Source: CAD feature listing. Evaluate the final solid. Frame: model axes, mm. A direction names the side the tool comes from. Give positions to 0.01 mm unless a question says otherwise; leave off trailing zeros. Write each loop counter-clockwise with the first axis right and the second up, starting at its lowest first coordinate (ties: lowest second). Pieces come first, ordered by that corner, then holes. Notation, with made-up numbers: (39, 79.5) - (68, 79.5) arc R29 ccw to (68, 99.5) - close; hole circle Ø1 at (71.25, -7.5). An arc over 180 degrees is marked (long way). Answer as a JSON object with one key per item and string values. Group by question number.
from build123d import *

# Parameters (mm, degrees)
F0_W        = 0.4
F0_H        = 28.4
F1_DEPTH    = 5
F2_T1_DEPTH = 17.9903810568
F3_T1_DEPTH = 29.4948974279
F3_T3_DEPTH = 30


# Not quite as in the source:
# - a fillet or chamfer that OpenCascade refuses, or shapes differently, is made with other operations: its cross-section is extruded or revolved along the edge and cut away or added


with BuildPart() as f1:
    # F0 (on Top) → F1 (new body)
    with BuildSketch(Plane.XY):
        Polygon((-17.5608190332, -5.5), (-10.5608190332, -5.5), (-11.8766345504, -2.5), (-14.2008190332, -2.5), (-14.2008190332, -0.1), (-14.2008190332, 0), (0, 0), (0, 28.4), (-6.4, 28.4), (-6.4, 26.9), (-2.4, 26.9), (-2.4, 2.7), (-12.7, 2.7), (-13.5608190332, 5.2), (-17.5608190332, 5.2), align=None)
        Polygon((-14.2008190332, 0), (-14.2008190332, -0.1), (0.4, -0.1), (0.4, 0), (0, 0), align=None)
        with Locations((0.2, 14.2)):
            Rectangle(F0_W, F0_H)
    extrude(amount=F1_DEPTH)

    # F2: fillet of radius 3 on 1 edges, made by hand

    # F2_s2 → F2_t1 (cut)
    with BuildSketch(Plane.XY.offset(-6.4951905284)):
        with BuildLine():
            ThreePointArc((-3.8019237886, 28.4), (-5.3019237886, 27.9980762114), (-6.4, 26.9))
            Line((-6.4, 26.9), (-6.4, 28.4))
            Line((-6.4, 28.4), (-3.8019237886, 28.4))
        make_face()
    extrude(amount=F2_T1_DEPTH, mode=Mode.SUBTRACT)

    # F3: fillet of radius 5 on 2 edges, made by hand

    # F3_s2 → F3_t1 (cut)
    with BuildSketch(Plane.XY.offset(-12.2474487139)):
        with BuildLine():
            ThreePointArc((-17.5608190332, 0.3010205144), (-16.4338023794, 3.4632981746), (-13.5608190332, 5.2))
            Line((-13.5608190332, 5.2), (-17.5608190332, 5.2))
            Line((-17.5608190332, 5.2), (-17.5608190332, 0.3010205144))
        make_face()
    extrude(amount=F3_T1_DEPTH, mode=Mode.SUBTRACT)

    # F3_s4 → F3_t3 (cut)
    with BuildSketch(Plane.XY.offset(-12.5)):
        with BuildLine():
            ThreePointArc((-17.5608190332, -0.5), (-16.0963529392, -4.0355339059), (-12.5608190332, -5.5))
            Line((-12.5608190332, -5.5), (-17.5608190332, -5.5))
            Line((-17.5608190332, -5.5), (-17.5608190332, -0.5))
        make_face()
    extrude(amount=F3_T3_DEPTH, mode=Mode.SUBTRACT)


solid = f1.part
Q1. Ray query, probe 1 along X at (y, z) = (15, 1.4); probe 2 along X at (y, z) = (3, 1.1); probe 3 along Y at (x, z) = (-3.25, 4.5). Return the intervals inside material, ascending. Write a range as [from, to].
Q2. Draft query along X for faces 1 (the cylindrical face through (-16.46, 3.43, 2.46)), 2 (the flat face through (-2, 8, 5)), 3 (the flat face through (0.4, 14, 2)), 4 (the flat face through (-13.124, 3.933, 2.465)). Return one class per face: released by +X, released by -X, zero draft, split by the parting line, or undercut.
Q3. First-contact query: pin 1 Ø1 at (x, z) = (-15, 1) entering from -Y; pin 2 Ø10 at (x, y) = (-7, 8) entering from -Z; pin 3 Ø1.5 at (x, y) = (-4.5, 4) entering from -Z; pin 4 Ø1.5 at (x, z) = (-9.5, 1.5) entering from -Y. Flat tips, straight axial feed; report the tip coordinate or a pass-through.
Q4. Section A-A on z = 3.05. Return the cut outline in (x, y), then the cut area to 3 significant figures.
Q5. Reachability of faces 5 (the flat face through (-4, 26.9, 2)), 6 (the flat face through (-11.21, -4.02, 2.46)), 7 (the flat face through (-7, 2.7, 2)) from +Z, -Z, +X, -X, +Y, -Y: full face, straight path, thin tool, end or side. Return the list, or none.
Q6. Section B-B on y = 10. Return the cut outline in (x, z), then the cut area to 3 significant figures.
Q7. Section C-C on x = -2. Return the cut outline in (y, z).
Taken from the geometry:
{
 "1": {"probe 1": "x = [-2.4, 0.4]", "probe 2": "x = [-16.77, -12.8], [-2.4, 0.4]", "probe 3": "y = [-0.1, 2.7], [26.9, 28.4]"},
 "2": {"face 1": "released by -X", "face 2": "zero draft", "face 3": "released by +X", "face 4": "undercut"},
 "3": {"pin 1": "stops at y = -5.11", "pin 2": "stops at z = 0", "pin 3": "passes through", "pin 4": "stops at y = -0.1"},
 "4": {"outline": "(-17.56, -0.5) arc R5 ccw to (-12.56, -5.5) - (-10.56, -5.5) - (-11.88, -2.5) - (-14.2, -2.5) - (-14.2, -0.1) - (0.4, -0.1) - (0.4, 28.4) - (-3.8, 28.4) arc R3 ccw to (-6.4, 26.9) - (-2.4, 26.9) - (-2.4, 2.7) - (-12.7, 2.7) - (-13.56, 5.2) arc R5 ccw to (-17.56, 0.3) - close", "area": "155 mm²"},
 "5": {"face 5": "+Z, -Z, -X", "face 6": "+Z, -Z, +X", "face 7": "+Z, -Z"},
 "6": {"outline": "(-2.4, 0) - (0.4, 0) - (0.4, 5) - (-2.4, 5) - close", "area": "14.0 mm²"},
 "7": {"outline": "(-0.1, 0) - (28.4, 0) - (28.4, 5) - (-0.1, 5) - close"}
}
